Check sheet for the drawn part. Datum: minimum x, y, z corner. Units: mm. A direction names the side the tool comes from. Give positions to 0.01 mm unless a question says otherwise; leave off trailing zeros. Order: outer loops, then holes, each group sorted by start corner. A loop starts at its lowest first (then second) coordinate and runs counter-clockwise, first axis right, second up. Notation, with made-up numbers: (45, 4) -> (75, 4) arc R22 cw to (75, 37) -> close; hole circle Ø2 at (63.25, -9). An arc over 180 degrees is marked (long way). Return JSON: item names as keys, results as strings. Group by question number.
(1) Cross-section at C-C on z = 15.25. Enter the section's corners in (x, y).
(2) Thickness scan on line 1 along Y through (x, z) = (27.5, 14); line 2 along Y through (x, z) = (26, 24.25); line 3 along X through (y, z) = (9, 28.25). Record the ranges inside material, lowest first.
(3) Tool access check on the marked faces 1 and 2. Record the directions out of +Z, -Z, +X, -X, +Y, -Y that give a thin tool (end or side, any length) a straight path to the whole face; none if there is none.
(4) Cross-section at A-A on y = 27.5. Enter the section's corners in (x, z).
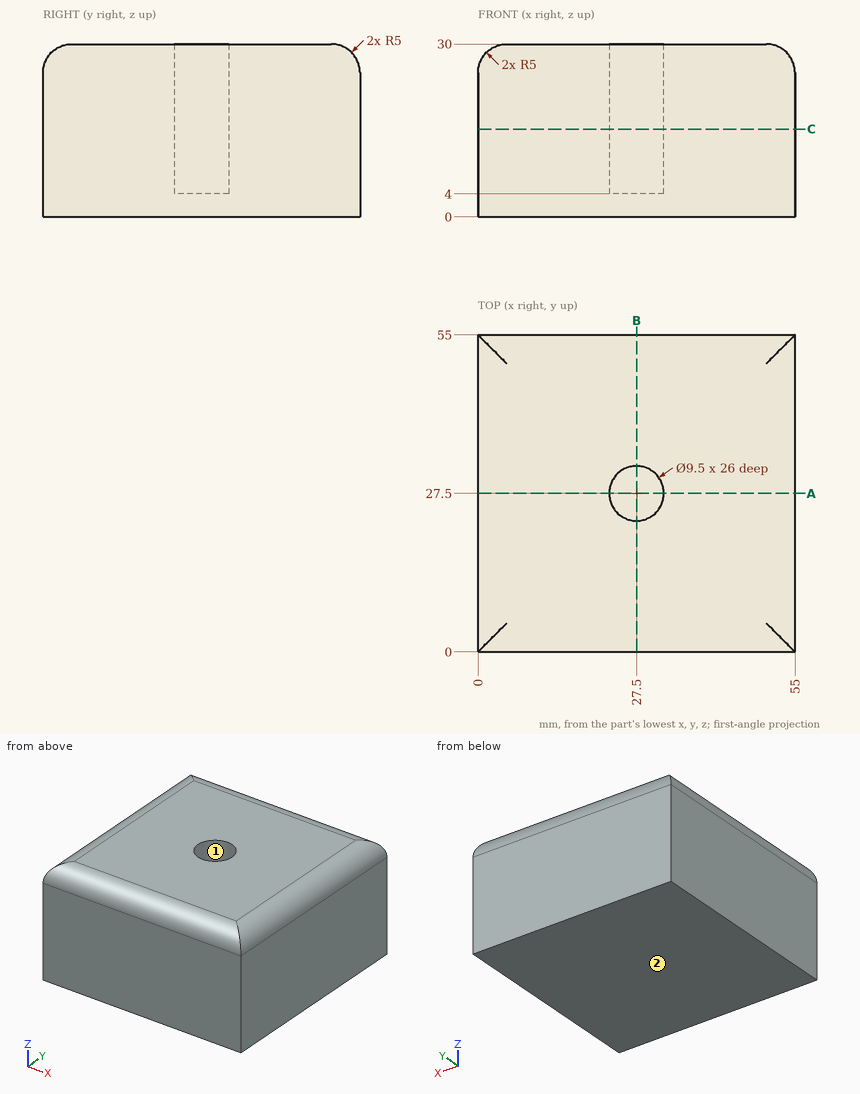
Verdict:
{
 "1": {"outline": "(0, 0) -> (55, 0) -> (55, 55) -> (0, 55) -> close; hole circle Ø9.5 at (27.5, 27.5)"},
 "2": {"line 1": "0 to 22.75, 32.25 to 55", "line 2": "0 to 22.99, 32.01 to 55", "line 3": "1.2 to 53.8"},
 "3": {"face 1": "+Z", "face 2": "-Z, +X, -X, +Y, -Y"},
 "4": {"outline": "(0, 0) -> (55, 0) -> (55, 25) arc R5 ccw to (50, 30) -> (32.25, 30) -> (32.25, 4) -> (22.75, 4) -> (22.75, 30) -> (5, 30) arc R5 ccw to (0, 25) -> close"}
}
